Can you work these out from the model? Positions are in its coordinate system, mm. Face numbers are marked on the shaded views. A direction names the side the tool comes from. Round coordinates to 2 decimals unless told otherwise and drop trailing zeros. Write each loop counter-clockwise with the first axis right and the second up, starting at its lowest first coordinate (ties: lowest second). Pieces come first, ordered by that corner, then holes. Notation, with made-up numbers: (-3.5, 59) -> (32.5, 59) arc R19 ccw to (32.5, 68) -> close; hole circle Ø2 at (9.25, 21). An arc over 180 degrees is marked (long way). Write item = value, one per line. Start each with the question number.
1) Thinking about a two-plate mould opening in Z: for the marked faces 1, 2 and 3, which applies, +Z half, -Z half, draft (parallel to the pull), parting line (faces both ways), or undercut?
2) For the marked faces 4 and 5, which set-ups out of +Z, -Z, +X, -X, +Y, -Y let a thin tool reach every point of the face, with its end or its side?
3) Imagine slicing it at B-B, the plane y = 11.5. Please give me the cut outline in (x, z) (1 decimal).
4) Imagine slicing it at A-A, the plane x = 20. Please give me the cut outline in (y, z) (1 decimal).
5) If I drill on line 1 (Z direction, x = 60.5, y = 4.5) (3 decimals); line 2 (X direction, y = 9.75, z = -11); line 3 (X direction, y = 12, z = -7), over which ranges is the centre line in solid material (lowest first)?
6) I'm going to push flat-ended pins straight in: pin 1 (7 mm diameter, centred on x = 46.5, z = -21.5, fed in from +Y); pin 2 (22.5 mm diameter, centred on x = 18.5, z = -21.5, fed in from +Y); pin 3 (3.5 mm diameter, centred on x = 31.88, z = -11.11, fed in from +Y). Where does each tip first touch, or does it pass through?
from build123d import *

# Parameters (mm, degrees)
SKETCH1_W             = 64.77
SKETCH1_H             = 40.005
BOSS_EXTRUDE1_DEPTH   = 15.494
CAVITY1_START         = 5.334
CAVITY1_OUTLINE_R     = 1.143
CAVITY1_OUTLINE_R_2   = 4.445
CAVITY1_DEPTH         = 10.16
CAVITY1_2_OUTLINE_R   = 1.143
CAVITY1_2_OUTLINE_R_2 = 7.239
CAVITY1_2_DEPTH       = 5.334
CAVITY1_START_2       = 2.286
CAVITY1_3_OUTLINE_R   = 4.445
CAVITY1_3_DEPTH       = 3.048
CAVITY1_START_3       = 13.716
CAVITY1_4_DEPTH       = 1.778
CAVITY1_5_OUTLINE_R   = 1.905
CAVITY1_5_OUTLINE_R_2 = 1.143
CAVITY1_5_DEPTH       = 3.302
CAVITY1_START_4       = 4.064
CAVITY1_6_OUTLINE_R   = 2.286
CAVITY1_6_DEPTH       = 1.27
CAVITY1_START_5       = 2.032
CAVITY1_7_DEPTH       = 0.254
SKETCH3_R             = 1.905
CUT_EXTRUDE1_DEPTH    = 6.35
FILLET1_R             = 1.5875


# Read off the part's stored shape, not the designer's step: Cavity1
with BuildPart() as part:
    # Sketch1 → Boss-Extrude1 (new body)
    with BuildSketch(Plane(origin=(0, 0, 0), x_dir=(1, 0, 0), z_dir=(0, 1, 0))):
        with Locations((32.385, 20.0025)):
            Rectangle(SKETCH1_W, SKETCH1_H)
    extrude(amount=BOSS_EXTRUDE1_DEPTH)

    # Cavity1 outline → Cavity1 (cut)
    with BuildSketch(Plane(origin=(0, 0, 0), x_dir=(1, 0, 0), z_dir=(0, 1, 0)).offset(CAVITY1_START)):
        with Locations((10.541, 6.0325)):
            Circle(CAVITY1_OUTLINE_R)
        with BuildLine():
            ThreePointArc((9.454432496, 9.938371148), (19.685, 5.6515), (29.915567504, 9.938371148))
            ThreePointArc((29.915567504, 9.938371148), (33.724105214, 9.765652448), (32.395188518, 13.338994253))
            ThreePointArc((32.395188518, 13.338994253), (34.036, 20.0025), (32.395188518, 26.666005747))
            ThreePointArc((32.395188518, 26.666005747), (33.724105214, 30.239347552), (29.915567504, 30.066628852))
            ThreePointArc((29.915567504, 30.066628852), (19.685, 34.3535), (9.454432496, 30.066628852))
            ThreePointArc((9.454432496, 30.066628852), (5.645894786, 30.239347552), (6.974811482, 26.666005747))
            ThreePointArc((6.974811482, 26.666005747), (5.334, 20.0025), (6.974811482, 13.338994253))
            ThreePointArc((6.974811482, 13.338994253), (5.645894786, 9.765652448), (9.454432496, 9.938371148))
        make_face()
        with Locations((54.229, 6.0325)):
            Circle(CAVITY1_OUTLINE_R)
        with Locations((45.085, 20.0025)):
            Circle(CAVITY1_OUTLINE_R_2)
        with Locations((10.541, 33.9725)):
            Circle(CAVITY1_OUTLINE_R)
        with Locations((54.229, 33.9725)):
            Circle(CAVITY1_OUTLINE_R)
    extrude(amount=CAVITY1_DEPTH, mode=Mode.SUBTRACT)

    # Cavity1 2 outline → Cavity1 2 (cut)
    with BuildSketch(Plane(origin=(0, 0, 0), x_dir=(1, 0, 0), z_dir=(0, 1, 0))):
        with Locations((10.541, 6.0325)):
            Circle(CAVITY1_2_OUTLINE_R)
        with Locations((54.229, 6.0325)):
            Circle(CAVITY1_2_OUTLINE_R)
        with Locations((10.541, 33.9725)):
            Circle(CAVITY1_2_OUTLINE_R)
        with Locations((54.229, 33.9725)):
            Circle(CAVITY1_2_OUTLINE_R)
        with Locations((19.685, 20.0025)):
            Circle(CAVITY1_2_OUTLINE_R_2)
    extrude(amount=CAVITY1_2_DEPTH, mode=Mode.SUBTRACT)

    # Cavity1 3 outline → Cavity1 3 (cut)
    with BuildSketch(Plane(origin=(0, 0, 0), x_dir=(1, 0, 0), z_dir=(0, 1, 0)).offset(CAVITY1_START_2)):
        with BuildLine():
            ThreePointArc((33.571815, 23.62293784), (28.575, 20.0025), (33.571815, 16.38206216))
            ThreePointArc((33.571815, 16.38206216), (34.036, 20.0025), (33.571815, 23.62293784))
        make_face()
        with Locations((45.085, 20.0025)):
            Circle(CAVITY1_3_OUTLINE_R)
    extrude(amount=CAVITY1_3_DEPTH, mode=Mode.SUBTRACT)

    # Cavity1 4 outline → Cavity1 4 (cut)
    with BuildSketch(Plane(origin=(0, 0, 0), x_dir=(1, 0, 0), z_dir=(0, 1, 0)).offset(CAVITY1_START_3)):
        with BuildLine():
            Line((44.074058668, 15.673987251), (45.983725966, 13.732738237))
            ThreePointArc((45.983725966, 13.732738237), (49.973349777, 14.396955949), (52.752669641, 17.335265738))
            Line((52.752669641, 17.335265738), (49.261068942, 18.479846661))
            ThreePointArc((49.261068942, 18.479846661), (47.1998806, 16.092857427), (44.074058668, 15.673987251))
        make_face()
        with BuildLine():
            ThreePointArc((40.766648336, 18.740599029), (42.59266679, 15.421456381), (45.983725966, 13.732738237))
            Line((45.983725966, 13.732738237), (44.074058668, 15.673987251))
            ThreePointArc((44.074058668, 15.673987251), (42.028662496, 16.774989185), (40.817941907, 18.757413564))
            Line((40.817941907, 18.757413564), (40.766648336, 18.740599029))
        make_face()
        with BuildLine():
            Line((49.261068942, 18.479846661), (52.752669641, 17.335265738))
            ThreePointArc((52.752669641, 17.335265738), (53.19142936, 18.636932759), (53.34, 20.0025))
            ThreePointArc((53.34, 20.0025), (53.19142936, 21.368067241), (52.752669641, 22.669734262))
            Line((52.752669641, 22.669734262), (49.261068942, 21.525153339))
            ThreePointArc((49.261068942, 21.525153339), (49.462250932, 20.775610132), (49.53, 20.0025))
            ThreePointArc((49.53, 20.0025), (49.462250932, 19.229389868), (49.261068942, 18.479846661))
        make_face()
        with BuildLine():
            ThreePointArc((40.704577582, 19.099192174), (40.73304351, 18.919450842), (40.766648336, 18.740599029))
            Line((40.766648336, 18.740599029), (40.817941907, 18.757413564))
            ThreePointArc((40.817941907, 18.757413564), (40.776510846, 18.909364048), (40.740488936, 19.062686925))
            Line((40.740488936, 19.062686925), (40.704577582, 19.099192174))
        make_face()
        with BuildLine():
            Line((49.261068942, 21.525153339), (52.752669641, 22.669734262))
            ThreePointArc((52.752669641, 22.669734262), (49.973349777, 25.608044051), (45.983725966, 26.272261763))
            Line((45.983725966, 26.272261763), (44.074058668, 24.33101275))
            ThreePointArc((44.074058668, 24.33101275), (47.1998806, 23.912142573), (49.261068942, 21.525153339))
        make_face()
        with BuildLine():
            Line((40.817941907, 21.247586436), (40.766648336, 21.264400971))
            ThreePointArc((40.766648336, 21.264400971), (40.73304351, 21.085549158), (40.704577582, 20.905807826))
            Line((40.704577582, 20.905807826), (40.740488936, 20.942313075))
            ThreePointArc((40.740488936, 20.942313075), (40.776510846, 21.095635952), (40.817941907, 21.247586436))
        make_face()
        with BuildLine():
            ThreePointArc((45.983725966, 26.272261763), (42.59266679, 24.583543619), (40.766648336, 21.264400971))
            Line((40.766648336, 21.264400971), (40.817941907, 21.247586436))
            ThreePointArc((40.817941907, 21.247586436), (42.028662496, 23.230010815), (44.074058668, 24.33101275))
            Line((44.074058668, 24.33101275), (45.983725966, 26.272261763))
        make_face()
        with BuildLine():
            ThreePointArc((40.64, 20.0025), (40.656164971, 19.549693393), (40.704577582, 19.099192174))
            Line((40.704577582, 19.099192174), (40.740488936, 19.062686925))
            ThreePointArc((40.740488936, 19.062686925), (40.665193631, 19.529914917), (40.64, 20.0025))
        make_face()
        with BuildLine():
            Line((40.740488936, 20.942313075), (40.704577582, 20.905807826))
            ThreePointArc((40.704577582, 20.905807826), (40.656164971, 20.455306607), (40.64, 20.0025))
            ThreePointArc((40.64, 20.0025), (40.665193631, 20.475085083), (40.740488936, 20.942313075))
        make_face()
    extrude(amount=CAVITY1_4_DEPTH, mode=Mode.SUBTRACT)

    # Cavity1 5 outline → Cavity1 5 (cut)
    # profile 1 of 4: a face of its own
    with BuildSketch(Plane(origin=(0, 0, 0), x_dir=(1, 0, 0), z_dir=(0, 1, 0))):
        with Locations((10.541, 6.0325)):
            Circle(CAVITY1_5_OUTLINE_R)
        with Locations((10.541, 6.0325)):
            Circle(CAVITY1_5_OUTLINE_R_2, mode=Mode.SUBTRACT)
    # profile 2 of 4: a face of its own
    with BuildSketch(Plane(origin=(0, 0, 0), x_dir=(1, 0, 0), z_dir=(0, 1, 0))):
        with Locations((54.229, 6.0325)):
            Circle(CAVITY1_5_OUTLINE_R)
        with Locations((54.229, 6.0325)):
            Circle(CAVITY1_5_OUTLINE_R_2, mode=Mode.SUBTRACT)
    # profile 3 of 4: a face of its own
    with BuildSketch(Plane(origin=(0, 0, 0), x_dir=(1, 0, 0), z_dir=(0, 1, 0))):
        with Locations((10.541, 33.9725)):
            Circle(CAVITY1_5_OUTLINE_R)
        with Locations((10.541, 33.9725)):
            Circle(CAVITY1_5_OUTLINE_R_2, mode=Mode.SUBTRACT)
    # profile 4 of 4: a face of its own
    with BuildSketch(Plane(origin=(0, 0, 0), x_dir=(1, 0, 0), z_dir=(0, 1, 0))):
        with Locations((54.229, 33.9725)):
            Circle(CAVITY1_5_OUTLINE_R)
        with Locations((54.229, 33.9725)):
            Circle(CAVITY1_5_OUTLINE_R_2, mode=Mode.SUBTRACT)
    extrude(amount=CAVITY1_5_DEPTH, mode=Mode.SUBTRACT)

    # Cavity1 6 outline → Cavity1 6 (cut)
    with BuildSketch(Plane(origin=(0, 0, 0), x_dir=(1, 0, 0), z_dir=(0, 1, 0)).offset(CAVITY1_START_4)):
        with Locations((7.493, 11.1125)):
            Circle(CAVITY1_6_OUTLINE_R)
        with Locations((31.877, 11.1125)):
            Circle(CAVITY1_6_OUTLINE_R)
        with Locations((7.493, 28.8925)):
            Circle(CAVITY1_6_OUTLINE_R)
        with Locations((31.877, 28.8925)):
            Circle(CAVITY1_6_OUTLINE_R)
    extrude(amount=CAVITY1_6_DEPTH, mode=Mode.SUBTRACT)

    # Cavity1 7 outline → Cavity1 7 (cut)
    with BuildSketch(Plane(origin=(0, 0, 0), x_dir=(1, 0, 0), z_dir=(0, 1, 0)).offset(CAVITY1_START_5)):
        with BuildLine():
            ThreePointArc((33.571815, 23.62293784), (28.575, 20.0025), (33.571815, 16.38206216))
            ThreePointArc((33.571815, 16.38206216), (34.036, 20.0025), (33.571815, 23.62293784))
        make_face()
    extrude(amount=CAVITY1_7_DEPTH, mode=Mode.SUBTRACT)

    # Sketch3 → Cut-Extrude1 (cut)
    with BuildSketch(Plane.XZ):
        with Locations(Location((4.7625, -35.2425, 0), (0, 0, 270))):
            Circle(SKETCH3_R)
        with Locations(Location((60.0075, -35.2425, 0), (0, 0, 270))):
            Circle(SKETCH3_R)
    cut_extrude1 = extrude(amount=-CUT_EXTRUDE1_DEPTH, mode=Mode.SUBTRACT)

    # Mirror3: Cut-Extrude1 across plane
    add(cut_extrude1.mirror(Plane(origin=(0, 0, -20.0025), x_dir=(1, 0, 0), z_dir=(0, 0, -1))), mode=Mode.SUBTRACT)

    # Fillet1
    fillet1_edges = [part.edges().sort_by_distance(p)[0] for p in [
        (64.77, 15.494, -20.0025),
        (32.385, 15.494, -40.005),
        (0, 15.494, -20.0025),
        (32.385, 0, -40.005),
        (64.77, 0, -20.0025),
        (32.385, 0, 0),
        (0, 0, -20.0025),
        (0, 7.747, -40.005),
        (64.77, 7.747, -40.005),
        (64.77, 7.747, 0),
        (0, 7.747, 0),
        (32.385, 15.494, 0),
    ]]
    fillet(fillet1_edges, radius=FILLET1_R)


solid = part.part
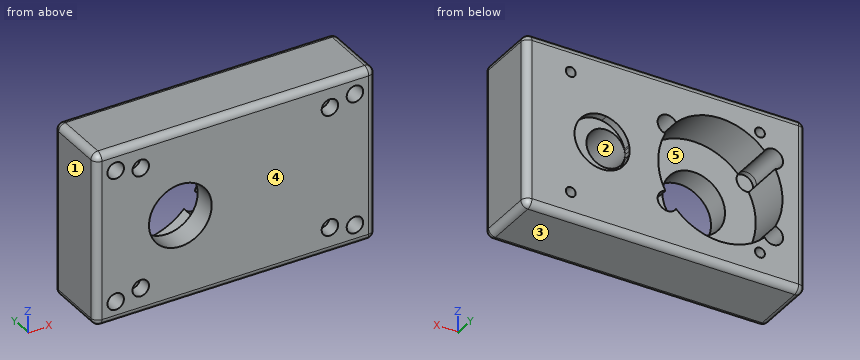
Reported:
q1.face_1 = draft
q1.face_2 = undercut
q1.face_3 = -Z half
q2.face_4 = +Z, -Z, +X, -X, -Y
q2.face_5 = +Y
q3.outline = (0, -38.4) arc R1.6 ccw to (1.6, -40) -> (63.2, -40) arc R1.6 ccw to (64.8, -38.4) -> (64.8, -1.6) arc R1.6 ccw to (63.2, 0) -> (1.6, 0) arc R1.6 ccw to (0, -1.6) -> close; hole (7, -26.7) arc R2.3 ccw (long way) to (9.5, -30.1) arc R14.4 ccw to (29.9, -30.1) arc R2.3 ccw (long way) to (32.4, -26.7) arc R14.4 ccw to (32.4, -13.3) arc R2.3 ccw (long way) to (29.9, -9.9) arc R14.4 ccw to (9.5, -9.9) arc R2.3 ccw (long way) to (7, -13.3) arc R14.4 ccw to start; hole circle Ø2.3 at (10.5, -34); hole circle Ø2.3 at (10.5, -6); hole circle Ø8.9 at (45.1, -20); hole circle Ø2.3 at (54.2, -34); hole circle Ø2.3 at (54.2, -6)
q4.outline = (0, -38.4) arc R1.6 ccw to (1.6, -40) -> (13.9, -40) arc R1.6 ccw to (15.5, -38.4) -> (15.5, -34.4) -> (5.3, -34.4) -> (5.3, -27.2) -> (0, -27.2) -> close; (0, -12.8) -> (5.3, -12.8) -> (5.3, -5.7) -> (15.5, -5.7) -> (15.5, -1.6) arc R1.6 ccw to (13.9, 0) -> (1.6, 0) arc R1.6 ccw to (0, -1.6) -> close
q5.line_1 = -40.005 to -37.083, -33.402 to -6.603, -2.922 to 0
q5.line_2 = 0 to 5.21, 34.16 to 64.77
q5.line_3 = 0 to 9.93, 11.15 to 13.61, 25.76 to 53.62, 54.84 to 64.77
q6.pin_1 = 13.72
q6.pin_2 = 5.33
q6.pin_3 = 4.06
